Input: part model. Units: mm. Frame: model coordinates. Give positions to 0.01 mm unless a question says otherwise; leave off trailing zeros. Loops run counter-clockwise (first coordinate to the right, second up) from the corner with the lowest first, then second, coordinate; pieces in that order, holes last. Notation, with made-up numbers: M 22.5,5 L 30.5,5 A12 cw 30.5,14 Z; hole C 53,65 d2. An arc over 180 degrees is marked long. Answer as a JSON object with one key per item and string values. Group by question number.
1) Section query B-B on y = 42.5. Return loops of the section in (x, z).
2) Ray query, L1, parallel to X at y = 17.5, z = 5.25. Return the intervals inside material, ascending.
3) Section query C-C on x = 27. Return loops of the section in (y, z), plus the area to 3 significant figures.
4) Section query A-A on z = 3.25. Return loops of the section in (x, y).
5) First-contact query: P1, Ø1.9, axis at y = 25.5, z = 2.5, coming from the +X side; P2, Ø12, axis at x = 185, y = 248, coming from the -Z side; P3, Ø1.9, axis at x = 32.5, z = 2.5, coming from the +Y side; P4, Ø1.9, axis at y = 278.5, z = 2.5, coming from the -X side. Flat tips, straight axial feed; report the tip coordinate or a pass-through.
Autodesk Fusion 360 part; units mm, degrees
sketch "Sketch1" plane through (0, 0, 0) normal (0, 0, 1) x (1, 0, 0)
  line L0 (0, 0) -> (0, 304.8)
  line L1 (0, 304.8) -> (304.8, 304.8)
  line L2 (304.8, 304.8) -> (304.8, 0)
  line L3 (304.8, 0) -> (0, 0)
  line L4 (0, 0) -> (50.8, 0)
  line L5 (50.8, 0) -> (50.8, 50.8)
  line L6 (50.8, 50.8) -> (0, 50.8)
  line L7 (0, 50.8) -> (0, 0)
  line L8 (0, 304.8) -> (50.8, 304.8)
  line L9 (50.8, 304.8) -> (50.8, 254)
  line L10 (50.8, 254) -> (0, 254)
  line L11 (0, 254) -> (0, 304.8)
  line L12 (304.8, 0) -> (298.45, 0)
  line L13 (298.45, 0) -> (298.45, 50.8)
  line L14 (298.45, 50.8) -> (304.8, 50.8)
  line L15 (304.8, 50.8) -> (304.8, 0)
  dimension "d2" = 304.8
  dimension "d3" = 304.8
  dimension "d10" = 50.8
  dimension "d13" = 50.8
  dimension "d14" = 6.35
  dimension "d17" = 50.8
extrude "Extrude1" add sketch "Sketch1" along normal blind 6.35 contours L0 L1 L2 L3 L5 L6 L9 L10 L13 L14
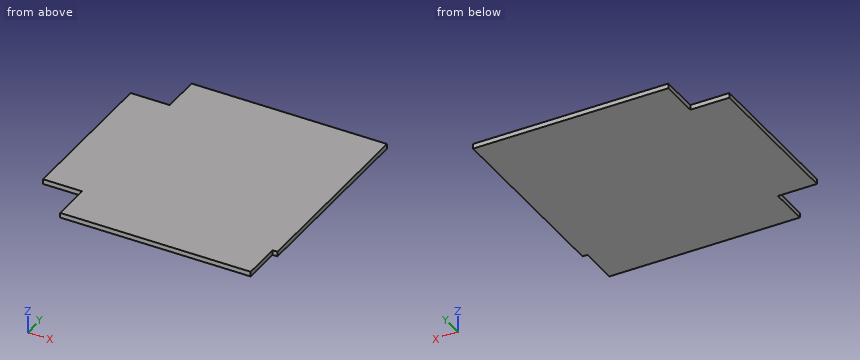
Output:
{
 "1": {"outline": "M 50.8,0 L 298.45,0 L 298.45,6.35 L 50.8,6.35 Z"},
 "2": {"L1": "x = 50.8 to 298.45"},
 "3": {"outline": "M 50.8,0 L 254,0 L 254,6.35 L 50.8,6.35 Z", "area": "1,290 mm^2"},
 "4": {"outline": "M 0,50.8 L 50.8,50.8 L 50.8,0 L 298.45,0 L 298.45,50.8 L 304.8,50.8 L 304.8,304.8 L 50.8,304.8 L 50.8,254 L 0,254 Z"},
 "5": {"P1": "stops at x = 298.45", "P2": "stops at z = 0", "P3": "stops at y = 254", "P4": "stops at x = 50.8"}
}
